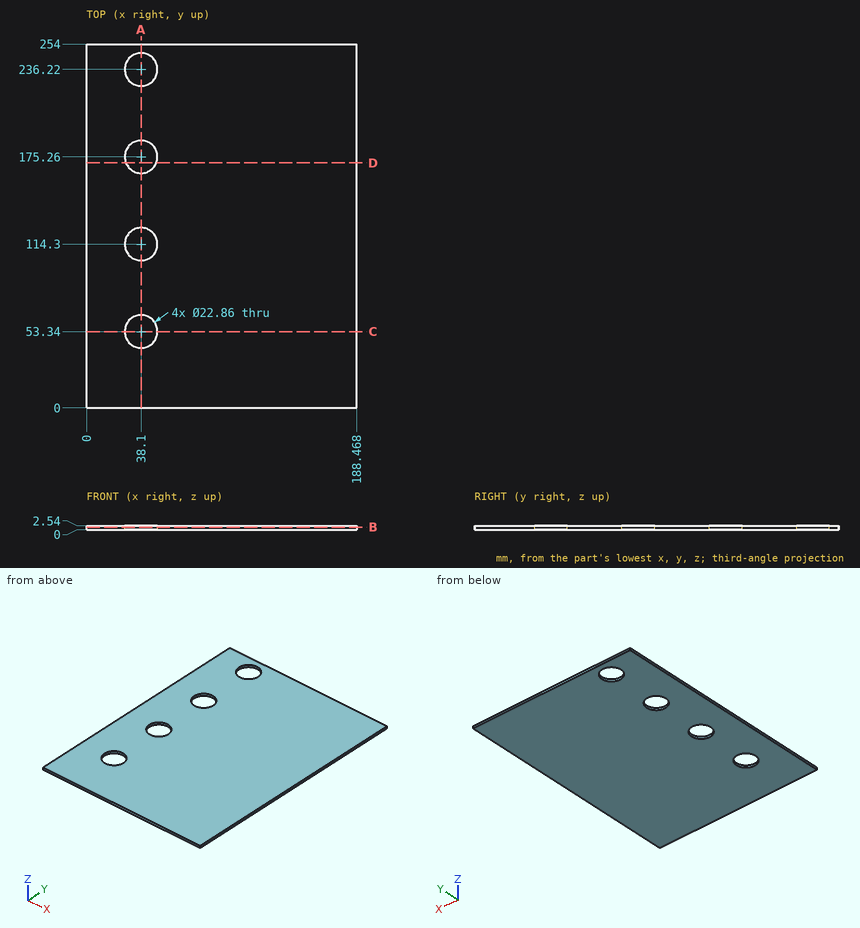
Input: dimensioned drawing with shaded views. Units: mm. Origin: part minimum x, y, z. Give positions to 0.01 mm unless a question says otherwise; leave off trailing zeros. Write each loop counter-clockwise with the first axis right and the second up, starting at its lowest first coordinate (ties: lowest second). Pieces come first, ordered by that corner, then holes. Notation, with made-up numbers: (38.5, 28.5) - (66.5, 28.5) arc R20 ccw to (66.5, 50.5) - close; hole circle Ø8 at (27, 66). An arc over 180 degrees is marked (long way). One line per item, written item: value. Start each with the question number.
Q1. Material intervals for probe 1 along Y at (x, z) = (38.1, 0.5); probe 2 along X at (y, z) = (175, 2.05); probe 3 along X at (y, z) = (106, 0.6), sorted ascending. Write a range as from..to.
Q2. Section query C-C, the plane y = 53.34. Return the cut outline in (x, z), then the cut area to 3 significant figures.
Q3. Section query B-B, the plane z = 1.65. Return the cut outline in (x, y).
Q4. Section query A-A, the plane x = 38.1. Return the cut outline in (y, z), then the cut area to 3 significant figures.
Q5. Section query D-D, the plane y = 171. Return the cut outline in (x, z), then the cut area to 3 significant figures.
Answer:
1. probe 1: y = 0..41.91, 64.77..102.87, 125.73..163.83, 186.69..224.79, 247.65..254
1. probe 2: x = 0..26.67, 49.53..188.47
1. probe 3: x = 0..30.24, 45.96..188.47
2. outline: (0, 0) - (26.67, 0) - (26.67, 2.54) - (0, 2.54) - close; (49.53, 0) - (188.47, 0) - (188.47, 2.54) - (49.53, 2.54) - close
2. area: 421 mm2
3. outline: (0, 0) - (188.47, 0) - (188.47, 254) - (0, 254) - close; hole circle Ø22.86 at (38.1, 53.34); hole circle Ø22.86 at (38.1, 114.3); hole circle Ø22.86 at (38.1, 175.26); hole circle Ø22.86 at (38.1, 236.22)
4. outline: (0, 0) - (41.91, 0) - (41.91, 2.54) - (0, 2.54) - close; (64.77, 0) - (102.87, 0) - (102.87, 2.54) - (64.77, 2.54) - close; (125.73, 0) - (163.83, 0) - (163.83, 2.54) - (125.73, 2.54) - close; (186.69, 0) - (224.79, 0) - (224.79, 2.54) - (186.69, 2.54) - close; (247.65, 0) - (254, 0) - (254, 2.54) - (247.65, 2.54) - close
4. area: 413 mm2
5. outline: (0, 0) - (27.49, 0) - (27.49, 2.54) - (0, 2.54) - close; (48.71, 0) - (188.47, 0) - (188.47, 2.54) - (48.71, 2.54) - close
5. area: 425 mm2
